Geometry check sheet. Reference: the model listing, model coordinates, mm. A direction names the side the tool comes from. Coordinates: 2 decimals unless noted, no trailing zeros. Order: outer loops, then holes, each group sorted by start corner. A loop starts at its lowest first (then second) coordinate and runs counter-clockwise, first axis right, second up. Notation, with made-up numbers: (74, 49.5) - (98, 49.5) arc R27 ccw to (98, 83.5) - close; hole circle Ø11 at (28.25, 40.5). An arc over 180 degrees is marked (long way). Put each result on its own line as item: value.
Autodesk Inventor part; units mm, degrees
ref_plane "YZ Plane" through (0, 0, 0) normal (1, 0, 0) x (0, 1, 0)
ref_plane "XZ Plane" through (0, 0, 0) normal (0, 1, 0) x (-1, 0, 0)
ref_plane "XY Plane" through (0, 0, 0) normal (0, 0, 1) x (1, 0, 0)
sketch "Sketch1" plane through (0, 0, 0) normal (0, 0, 1) x (1, 0, 0)
  line L0 (-27.5, 24.6716) -> (21.8431, -24.6716)
  line L1 (31.5, -28.6716) -> (-27.5, 30.3284)
  line L2 (-27.5, 30.3284) -> (-31.5, 30.3284)
  line L3 (31.5, -28.6716) -> (-31.5, -28.6716)
  line L4 (-27.5, -24.6716) -> (21.8431, -24.6716)
  line L5 (-27.5, 24.6716) -> (-27.5, -24.6716)
  line L6 (-31.5, 15.3284) -> (-51.5, 15.3284)
  line L7 (-51.5, 15.3284) -> (-51.5, 11.3284)
  line L8 (-51.5, 11.3284) -> (-31.5, 11.3284)
  line L9 (-31.5, 30.3284) -> (-31.5, 15.3284)
  line L10 (-31.5, 11.3284) -> (-31.5, -28.6716)
  point P0 (0, 0)
  point P1 (-27.5, 0)
  point P2 (0, -28.6716)
  dimension "d0" = 4
  dimension "d19" = 4
  dimension "d22" = 20
  dimension "d23" = 4
  dimension "d25" = 45
  dimension "d28" = 83.4386
  dimension "d29" = 4
  dimension "d30" = 4
  dimension "d35" = 40
extrude "Extrusion1" add sketch "Sketch1" along normal mid plane 8
sketch "Sketch5" plane through (-51.5, 15.3284, -4) normal (0, 1, 0) x (1, 0, 0)
  line L0 (20, -8) -> (20, 0)
  line L1 (0, 0) -> (20, 0)
  line L2 (0, -8) -> (0, 0)
  line L3 (20, -8) -> (0, -8)
  circle A0 centre (10, -4) radius 2.1
  point P0 (51.5, -4)
  point P1 (0, -4)
  dimension "d31" = 4.2
  dimension "d32" = 10
extrude "Extrusion4" cut sketch "Sketch5" against normal through all contours A0
sketch "Sketch6" plane through (-27.5, 30.3284, -4) normal (0.7071, 0.7071, 0) x (-0.7071, 0.7071, 0)
  circle A0 centre (-13.9386, 4) radius 1.6
  circle A1 centre (-63.4386, 4) radius 1.6
  line L0 (-83.4386, 0) -> (-83.4386, 8)
  point P0 (-40.8909, 4)
  point P1 (-83.4386, 4)
  dimension "d36" = 49.5
  dimension "d37" = 20
  dimension "d38" = 3.2
extrude "Extrusion5" cut sketch "Sketch6" against normal blind 6
sketch "Sketch7" plane through (0, 0, 4) normal (0, 0, 1) x (1, 0, 0)
  line L0 (31.5, -28.6716) -> (-27.5, 30.3284)
  line L1 (-31.5, -28.6716) -> (31.5, -28.6716)
  line L2 (28.6716, -25.8431) -> (25.8431, -28.6716)
  line L3 (25.8431, -28.6716) -> (31.5, -28.6716)
  line L4 (28.6716, -25.8431) -> (31.5, -28.6716)
  point P0 (0, 0)
  dimension "d42" = 4
extrude "Extrusion6" cut sketch "Sketch7" against normal through all
fillet "Fillet1" radius 2 5 edges at (-27.5, -24.6716, 0) (-27.5, 30.3284, 0) (28.6716, -25.8431, 0) (21.8431, -24.6716, 0) (-27.5, 24.6716, 0)
properties part number "holder-LCD-v2"
Q1. Depth check by flat-ended pin: pin 1 Ø2.5 at (x, z) = (-38.5, 1) entering from -Y; pin 2 Ø4 at (x, z) = (1.5, 0) entering from +Y; pin 3 Ø3 at (y, z) = (8.5, -3) entering from -X. Enter the tip coordinate at first touch or a pass-through.
Answer block:
pin 1: stops at y = 11.33
pin 2: stops at y = 3.33
pin 3: stops at x = -31.5
Q2. Thickness scan on L1, parallel to X at y = 12.45, z = 0; L2, parallel to X at y = 14.1, z = 0; L3, parallel to Y at x = -37, z = 1.25. Record the ranges inside material, lowest first. Write a range as [from, to].
Answer block:
L1: x = [-51.5, -43.6], [-39.4, -27.5], [-15.28, -9.62]
L2: x = [-51.5, -43.6], [-39.4, -27.5], [-16.93, -11.27]
L3: y = [11.33, 15.33]
Q3. Section check B-B on z = -3. Record the boundary of the cut face in (x, y).
Answer block:
outline: (-51.5, 11.33) - (-31.5, 11.33) - (-31.5, -28.67) - (25.84, -28.67) - (27.26, -27.26) arc R2 ccw to (27.26, -24.43) - (-26.91, 29.74) arc R2 ccw to (-28.33, 30.33) - (-31.5, 30.33) - (-31.5, 15.33) - (-51.5, 15.33) - close; hole (-27.5, -22.67) arc R2 ccw to (-25.5, -24.67) - (17.01, -24.67) arc R2 ccw to (18.43, -21.26) - (-24.09, 21.26) arc R2 ccw to (-27.5, 19.84) - close
Q4. Section check A-A on x = -41.5. Record the boundary of the cut face in (y, z), then the cut area to 3 significant figures.
Answer block:
outline: (11.33, -4) - (15.33, -4) - (15.33, -2.1) - (11.33, -2.1) - close; (11.33, 2.1) - (15.33, 2.1) - (15.33, 4) - (11.33, 4) - close
area: 15.2 mm^2
Q5. Access from +Z, -Z, +X, -X, +Y, -Y to the whole of each face (thin tool, end or side, straight path). Record for faces 1 (the flat face through (-44, 11.328, 0)), 2 (the flat face through (-5, -24.672, 0)), 3 (the flat face through (-39, 15.328, 0)).
Answer block:
face 1: +Z, -Z, -X, -Y
face 2: +Z, -Z
face 3: +Z, -Z, -X, +Y
Q6. Draft check along Z on faces 4 (the flat face through (-30, 30.328, 0)), 5 (the cylindrical face through (-20.117, 20.157, 0.481)), 6 (the flat face through (-3, 3, 4)). Enter one of: pulls with the +Z half, pulls with the -Z half, needs draft (parallel to the pull), parting line crosses it, or undercut.
Answer block:
face 4: needs draft
face 5: undercut
face 6: pulls with the +Z half
Q7. Section check D-D on y = 25.5. Record the boundary of the cut face in (x, z), then the cut area to 3 significant figures.
Answer block:
outline: (-31.5, -4) - (-22.67, -4) - (-22.67, 4) - (-31.5, 4) - close
area: 70.6 mm^2
Q8. Section check C-C on y = -23.5. Record the boundary of the cut face in (x, z), then the cut area to 3 significant figures.
Answer block:
outline: (-31.5, -4) - (-27.32, -4) - (-27.32, 4) - (-31.5, 4) - close; (18.84, -4) - (26.33, -4) - (26.33, 4) - (18.84, 4) - close
area: 93.4 mm^2
